```python
from build123d import *

# Parameters (mm, degrees)
BOSS_EXTRUDE1_DEPTH = 15
BOSS_EXTRUDE2_DEPTH = 365


with BuildPart() as part:
    # Sketch1 → Boss-Extrude1 (new body)
    with BuildSketch(Plane.XY):
        with BuildLine():
            Line((0, 0), (45.50587847, 169.830250493))
            ThreePointArc((45.50587847, 169.830250493), (59.224787839, 194.836520244), (82.940219448, 210.682665034))
            Line((82.940219448, 210.682665034), (162.723089982, 239.721255113))
            ThreePointArc((162.723089982, 239.721255113), (183.503155924, 252.5803501), (197.43217259, 272.658944651))
            Line((197.43217259, 272.658944651), (230.064782718, 349.536556424))
            ThreePointArc((230.064782718, 349.536556424), (248.493176125, 371.694291103), (276.090025391, 380))
            Line((276.090025391, 380), (311.040765772, 380))
            ThreePointArc((311.040765772, 380), (343.180146256, 368.302222156), (360.281153423, 338.682408883))
            Line((360.281153423, 338.682408883), (420, 0))
            Line((420, 0), (350, 0))
            Line((350, 0), (330.381422238, 28.018232726))
            ThreePointArc((330.381422238, 28.018232726), (303.576164909, 51.525812488), (268.945018916, 60))
            Line((268.945018916, 60), (151.054981084, 60))
            ThreePointArc((151.054981084, 60), (116.423835091, 51.525812488), (89.618577762, 28.018232726))
            Line((89.618577762, 28.018232726), (70, 0))
            Line((70, 0), (0, 0))
        make_face()
        with BuildLine():
            Line((268.565395581, 342.5), (318.565395581, 342.5))
            ThreePointArc((318.565395581, 342.5), (331.065395581, 330), (318.565395581, 317.5))
            Line((318.565395581, 317.5), (268.565395581, 317.5))
            ThreePointArc((268.565395581, 317.5), (256.065395581, 330), (268.565395581, 342.5))
        make_face(mode=Mode.SUBTRACT)
    boss_extrude1 = extrude(amount=BOSS_EXTRUDE1_DEPTH)

    # Sketch3 → Boss-Extrude2 (add)
    with BuildSketch(Plane.XY.offset(15)):
        Polygon((200, 115), (202.5, 115), (202.5, 130), (57.5, 130), (57.5, 115), (60, 115), (60, 80), (200, 80), align=None)
        Polygon((177.5, 220), (322.5, 220), (322.5, 205), (320, 205), (320, 170), (180, 170), (180, 205), (177.5, 205), align=None)
    extrude(amount=BOSS_EXTRUDE2_DEPTH)

    # Mirror1: Boss-Extrude1 across plane
    add(boss_extrude1.mirror(Plane.XY.offset(197.5)))


solid = part.part
```
Read the model definition and answer for the solid it produces. Units are mm, in the model's axes. A direction names the side the tool comes from. Coordinates: 2 decimals unless noted, no trailing zeros. Loops run counter-clockwise (first coordinate to the right, second up) from the corner with the lowest first, then second, coordinate; pieces in that order, holes last. Notation, with made-up numbers: (26, 6) - (39, 6) arc R14 ccw to (39, 16) - close; hole circle Ø2 at (32, -15). An arc over 180 degrees is marked (long way). Answer in a Markdown table with one row per item.
1. Find section B-B, the plane y = 254.5. Write down the section's boundary in (x, z).
Conclusion:
| item | result |
|---|---|
| outline | (185.44, 0) - (375.12, 0) - (375.12, 15) - (185.44, 15) - close; (185.44, 380) - (375.12, 380) - (375.12, 395) - (185.44, 395) - close |
2. Which of the six approach directions +Z, -Z, +X, -X, +Y, -Y give full straight-line access (tool end or side, diameter ignored) to faces 5 (the face through (340.33, 13.81, 387.6)), 6 (the face through (22.434, 83.726, 387.605)), 7 (the face through (320, 188, 195))?
Conclusion:
| item | result |
|---|---|
| face 5 | +Z, -Z, -Y |
| face 6 | +Z, -Z, -X, +Y |
| face 7 | +X, -Y |
3. Find section C-C, the plane y = 330. Write down the section's boundary in (x, z).
Conclusion:
| item | result |
|---|---|
| outline | (221.77, 0) - (256.07, 0) - (256.07, 15) - (221.77, 15) - close; (221.77, 380) - (256.07, 380) - (256.07, 395) - (221.77, 395) - close; (331.07, 0) - (361.81, 0) - (361.81, 15) - (331.07, 15) - close; (331.07, 380) - (361.81, 380) - (361.81, 395) - (331.07, 395) - close |
4. Find section A-A, the plane z = 259.5. Write down the section's boundary in (x, y), then the cut area to 4 significant figures.
Conclusion:
| item | result |
|---|---|
| outline | (57.5, 115) - (60, 115) - (60, 80) - (200, 80) - (200, 115) - (202.5, 115) - (202.5, 130) - (57.5, 130) - close; (177.5, 205) - (180, 205) - (180, 170) - (320, 170) - (320, 205) - (322.5, 205) - (322.5, 220) - (177.5, 220) - close |
| area | 14,150 mm² |
5. Given pin 1 (1 mm diameter, centred on x = 297, z = 263, fed in from -Y); pin 2 (3 mm diameter, centred on x = 178.5, z = 285.5, fed in from -Y); pin 3 (3 mm diameter, centred on x = 307.5, z = 184.5, fed in from +Y), each flat-ended and moving along its own axis, determine where each tip first touches the part or whether it passes through.
Conclusion:
| item | result |
|---|---|
| pin 1 | stops at y = 170 |
| pin 2 | stops at y = 80 |
| pin 3 | stops at y = 220 |
6. Find section D-D, the plane x = 76.5. Write down the section's boundary in (y, z).
Conclusion:
| item | result |
|---|---|
| outline | (9.28, 0) - (207.9, 0) - (207.9, 15) - (130, 15) - (130, 380) - (207.9, 380) - (207.9, 395) - (9.28, 395) - (9.28, 380) - (80, 380) - (80, 15) - (9.28, 15) - close |
7. Straight lines are drawn through the part: line 1 (Z direction, x = 340.5, y = 142); line 2 (Y direction, x = 266.5, z = 51); line 3 (Y direction, x = 196, z = 195). For each, find the intervals that lie inside material, in ascending order.
Conclusion:
| item | result |
|---|---|
| line 1 | z = 0 to 15, 380 to 395 |
| line 2 | y = 170 to 220 |
| line 3 | y = 80 to 130, 170 to 220 |
8. Determine the mould class of faces 1 (the face through (256.07, 329.73, 387.6)), 2 (the face through (294, 317.5, 388)), 3 (the face through (213.52, 310.56, 387.6)), 4 (the face through (213, 150, 0)) for opening direction Y: +Y half, -Y half, draft (parallel to the pull), parting line (faces both ways), or undercut.
Conclusion:
| item | result |
|---|---|
| face 1 | undercut |
| face 2 | undercut |
| face 3 | +Y half |
| face 4 | draft |
